Verification items for this drawing (mm, ordinates from the low corner). Give positions to 0.01 mm unless a question says otherwise; leave off trailing zeros. Loops run counter-clockwise (first coordinate to the right, second up) from the corner with the lowest first, then second, coordinate; pieces in that order, holes last. Notation, with made-up numbers: (27, 43.5) - (44, 43.5) arc R21 ccw to (44, 75.5) - close; hole circle Ø9 at (28.25, -10.5). An arc over 180 degrees is marked (long way). One line per question, with ' | ' between items. Start each with the question number.
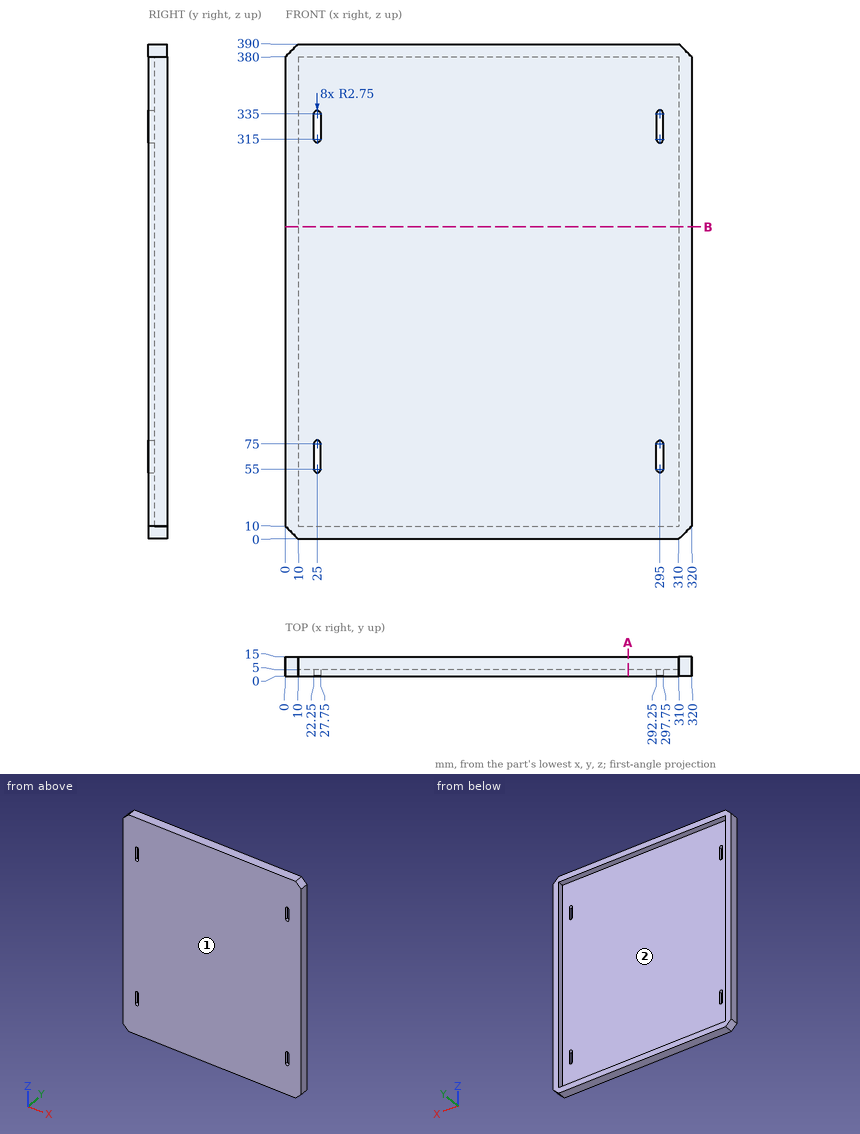
(1) Material ranges on line 1 (Z direction, x = 200, y = 7.75); line 2 (X direction, y = 13.5, z = 201); line 3 (Y direction, x = 116, z = 100), recorded low to high.
(2) Section check A-A, the plane x = 270. Record the boundary of the cut face in (y, z).
(3) Mould release check, pull along X, two halves, no side actions. Record for the marked faces 1 and 2: pulls with the +X half, pulls with the -X half, needs draft (parallel to the pull), parting line crosses it, or undercut.
(4) Section check B-B, the plane z = 246. Record the boundary of the cut face in (x, y), and give its area (3 significant figures).
Numbers:
1) line 1: 0 to 10, 380 to 390 | line 2: 0 to 10, 310 to 320 | line 3: 0 to 5
2) outline: (0, 0) - (15, 0) - (15, 10) - (5, 10) - (5, 380) - (15, 380) - (15, 390) - (0, 390) - close
3) face 1: needs draft | face 2: undercut
4) outline: (0, 0) - (320, 0) - (320, 15) - (310, 15) - (310, 5) - (10, 5) - (10, 15) - (0, 15) - close | area: 1,800 mm^2
